Print and shaded views of the part. All mm, measured from the part's lowest x, y and z. Coordinates: 2 decimals unless noted, no trailing zeros. Order: outer loops, then holes, each group sorted by start corner. A loop starts at its lowest first (then second) coordinate and runs counter-clockwise, first axis right, second up. Notation, with made-up numbers: (12, 45) -> (42, 45) arc R20 cw to (42, 78) -> close; hole circle Ø6 at (72.25, 49.5). An arc over 180 degrees is marked (long way). Write item = value, one per line. Start each with the question number.
Q1. Cut at A-A, the plane y = 133.35. List the corners of the cut face in (x, z).
Q2. Wall check: line 1 (Y direction, x = 6.35, z = 0.35); line 2 (X direction, y = 133.35, z = 1.25); line 3 (X direction, y = 6.35, z = 1.15). Give the ranges that are in metal, low to high. Write a range as from..to.
Q3. Cut at C-C, the plane x = 6.35. List the corners of the cut face in (y, z).
Q4. Cut at B-B, the plane z = 0.65. List the corners of the cut face in (x, y).
Q5. Cut at D-D, the plane y = 6.35. List the corners of the cut face in (x, z).
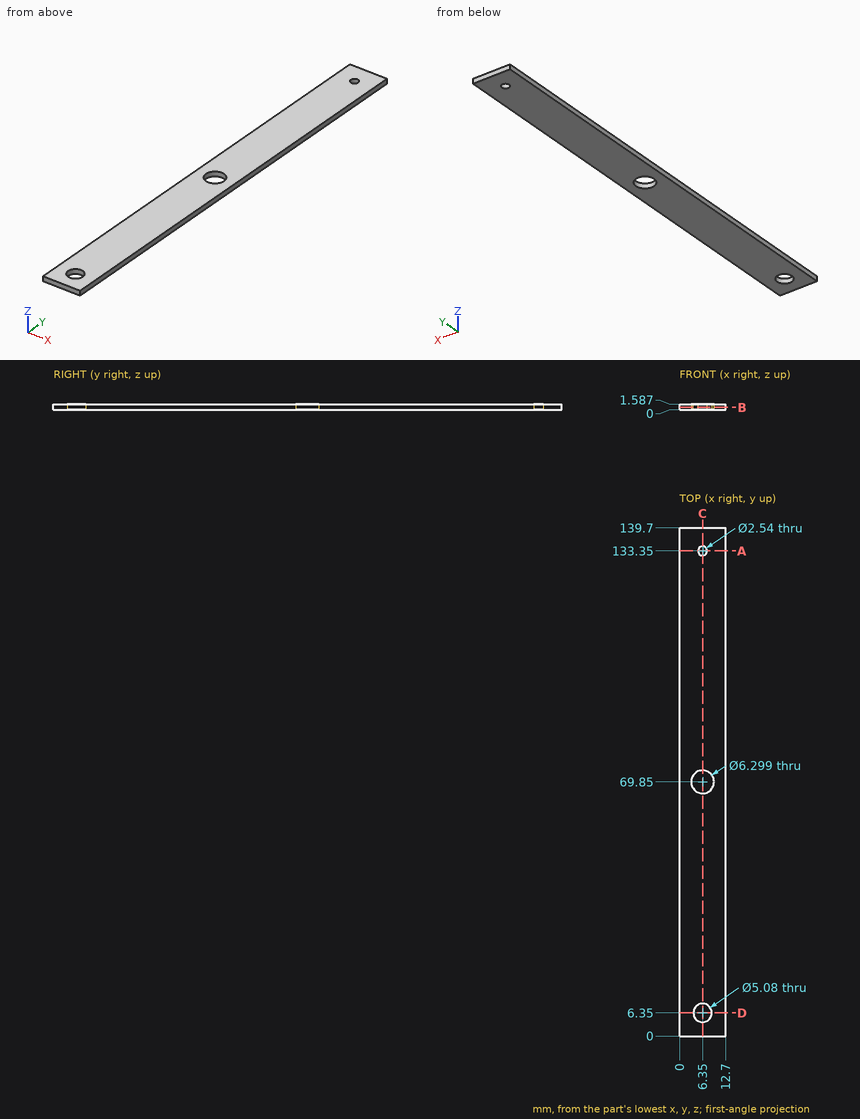
Here are the results:
q1.outline = (0, 0) -> (5.08, 0) -> (5.08, 1.59) -> (0, 1.59) -> close; (7.62, 0) -> (12.7, 0) -> (12.7, 1.59) -> (7.62, 1.59) -> close
q2.line_1 = 0..3.81, 8.89..66.7, 73..132.08, 134.62..139.7
q2.line_2 = 0..5.08, 7.62..12.7
q2.line_3 = 0..3.81, 8.89..12.7
q3.outline = (0, 0) -> (3.81, 0) -> (3.81, 1.59) -> (0, 1.59) -> close; (8.89, 0) -> (66.7, 0) -> (66.7, 1.59) -> (8.89, 1.59) -> close; (73, 0) -> (132.08, 0) -> (132.08, 1.59) -> (73, 1.59) -> close; (134.62, 0) -> (139.7, 0) -> (139.7, 1.59) -> (134.62, 1.59) -> close
q4.outline = (0, 0) -> (12.7, 0) -> (12.7, 139.7) -> (0, 139.7) -> close; hole circle Ø6.3 at (6.35, 69.85); hole circle Ø5.08 at (6.35, 6.35); hole circle Ø2.54 at (6.35, 133.35)
q5.outline = (0, 0) -> (3.81, 0) -> (3.81, 1.59) -> (0, 1.59) -> close; (8.89, 0) -> (12.7, 0) -> (12.7, 1.59) -> (8.89, 1.59) -> close
